Source: CAD feature listing. Evaluate the final solid. Frame: model axes, mm. Face numbers are marked on the shaded views. A direction names the side the tool comes from. Give positions to 0.01 mm unless a question says otherwise; leave off trailing zeros. Loops run counter-clockwise (first coordinate to the right, second up) from the corner with the lowest first, then second, coordinate; pieces in that order, holes last. Notation, with made-up numbers: (89, 78.5) -> (108, 78.5) arc R15 cw to (108, 105.5) -> close; hole circle Ø2 at (75, -4). An arc over 180 degrees is marked (long way). Answer as a JSON object with one key per item and string values. Group by question number.
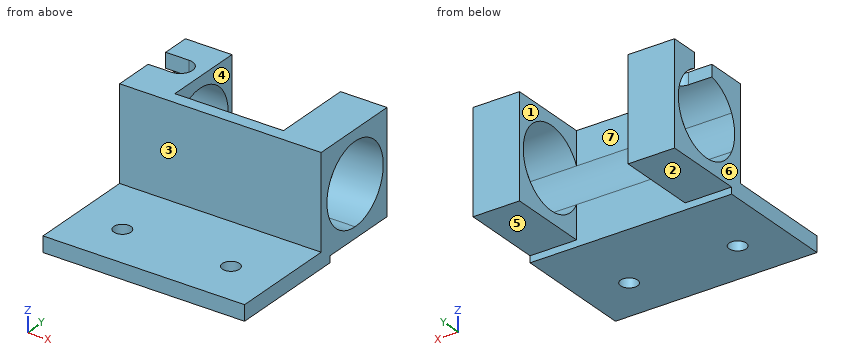
from build123d import *

# Parameters (mm, degrees)
CROQUIS2_W              = 65
CROQUIS2_H              = 35
CROQUIS2_R              = 2.75
SALIENTE_EXTRUIR1_DEPTH = 5
CROQUIS3_W              = 65
CROQUIS3_H              = 35
SALIENTE_EXTRUIR2_DEPTH = 4
SALIENTE_EXTRUIR3_DEPTH = 15
SALIENTE_EXTRUIR4_START = -65
SALIENTE_EXTRUIR4_DEPTH = 15
CORTAR_EXTRUIR1_DEPTH   = 85.965620518
CORTAR_EXTRUIR2_START   = -32.882450487
CORTAR_EXTRUIR2_DEPTH   = 4.823037372


# Read off the part's stored shape, not the designer's step: Cortar-Extruir2
with BuildPart() as part:
    # Croquis2 → Saliente-Extruir1 (new body)
    with BuildSketch(Plane.XY):
        with Locations((0, -5.5)):
            Rectangle(CROQUIS2_W, CROQUIS2_H)
        with Locations((17.5, -8)):
            Circle(CROQUIS2_R, mode=Mode.SUBTRACT)
        with Locations((-17.5, -8)):
            Circle(CROQUIS2_R, mode=Mode.SUBTRACT)
    extrude(amount=SALIENTE_EXTRUIR1_DEPTH)

    # Croquis3 → Saliente-Extruir2 (add)
    with BuildSketch(Plane(origin=(0, 12, 0), x_dir=(1, 0, 0), z_dir=(0, 1, 0))):
        with Locations((0, -17.5)):
            Rectangle(CROQUIS3_W, CROQUIS3_H)
    extrude(amount=SALIENTE_EXTRUIR2_DEPTH)

    # Croquis4 → Saliente-Extruir3 (add)
    with BuildSketch(Plane(origin=(32.5, 0, 0), x_dir=(0, 0, -1), z_dir=(1, 0, 0))):
        with BuildLine():
            Line((-35, 42.06134413), (-35, 16))
            Line((-35, 16), (-24.382874813, 16))
            ThreePointArc((-24.382874813, 16), (-25.295997358, 38.453973796), (-5.683774756, 27.482398858))
            ThreePointArc((-5.683774756, 27.482398858), (-7.587199819, 20.745176256), (-12.7346747, 16))
            Line((-12.7346747, 16), (-2.117549513, 16))
            Line((-2.117549513, 16), (-2.117549513, 42.06134413))
            Line((-2.117549513, 42.06134413), (-35, 42.06134413))
        make_face()
        with BuildLine():
            Line((-12.7346747, 16), (-24.382874813, 16))
            ThreePointArc((-24.382874813, 16), (-18.558774756, 14.607398858), (-12.7346747, 16))
        make_face()
        with BuildLine():
            ThreePointArc((-5.683774756, 27.482398858), (-25.295997358, 38.453973796), (-24.382874813, 16))
            Line((-24.382874813, 16), (-12.7346747, 16))
            ThreePointArc((-12.7346747, 16), (-7.587199819, 20.745176256), (-5.683774756, 27.482398858))
        make_face()
    extrude(amount=-SALIENTE_EXTRUIR3_DEPTH)

    # Croquis4<6> → Saliente-Extruir4 (add)
    with BuildSketch(Plane(origin=(32.5, 0, 0), x_dir=(0, 0, -1), z_dir=(1, 0, 0)).offset(SALIENTE_EXTRUIR4_START)):
        with BuildLine():
            Line((-35, 42.06134413), (-35, 16))
            Line((-35, 16), (-24.382874813, 16))
            ThreePointArc((-24.382874813, 16), (-25.295997358, 38.453973796), (-5.683774756, 27.482398858))
            ThreePointArc((-5.683774756, 27.482398858), (-7.587199819, 20.745176256), (-12.7346747, 16))
            Line((-12.7346747, 16), (-2.117549513, 16))
            Line((-2.117549513, 16), (-2.117549513, 42.06134413))
            Line((-2.117549513, 42.06134413), (-35, 42.06134413))
        make_face()
        with BuildLine():
            Line((-12.7346747, 16), (-24.382874813, 16))
            ThreePointArc((-24.382874813, 16), (-18.558774756, 14.607398858), (-12.7346747, 16))
        make_face()
        with BuildLine():
            ThreePointArc((-5.683774756, 27.482398858), (-25.295997358, 38.453973796), (-24.382874813, 16))
            Line((-24.382874813, 16), (-12.7346747, 16))
            ThreePointArc((-12.7346747, 16), (-7.587199819, 20.745176256), (-5.683774756, 27.482398858))
        make_face()
    extrude(amount=SALIENTE_EXTRUIR4_DEPTH)

    # Croquis4<4> → Cortar-Extruir1 (cut, through all)
    with BuildSketch(Plane(origin=(32.5, 0, 0), x_dir=(0, 0, -1), z_dir=(1, 0, 0))):
        with BuildLine():
            Line((-12.7346747, 16), (-24.382874813, 16))
            ThreePointArc((-24.382874813, 16), (-18.558774756, 14.607398858), (-12.7346747, 16))
        make_face()
        with BuildLine():
            ThreePointArc((-5.683774756, 27.482398858), (-25.295997358, 38.453973796), (-24.382874813, 16))
            Line((-24.382874813, 16), (-12.7346747, 16))
            ThreePointArc((-12.7346747, 16), (-7.587199819, 20.745176256), (-5.683774756, 27.482398858))
        make_face()
    extrude(amount=-CORTAR_EXTRUIR1_DEPTH, mode=Mode.SUBTRACT)

    # Cortar-Extruir2 outline → Cortar-Extruir2 (cut)
    with BuildSketch(Plane(origin=(0, 0, 2.117549513), x_dir=(-1, 0, 0), z_dir=(0, 0, -1)).offset(CORTAR_EXTRUIR2_START)):
        with BuildLine():
            Line((32.5, 33.030672065), (25, 33.030672065))
            ThreePointArc((25, 33.030672065), (21, 29.030672065), (25, 25.030672065))
            Line((25, 25.030672065), (32.5, 25.030672065))
            Line((32.5, 25.030672065), (32.5, 33.030672065))
        make_face()
    extrude(amount=CORTAR_EXTRUIR2_DEPTH, mode=Mode.SUBTRACT)


solid = part.part
(1) Material intervals for line 1 (X direction, y = 16.5, z = 31.5); line 2 (Z direction, x = -8, y = 5); line 3 (Y direction, x = 0, z = 25), sorted ascending. Write a range as from..to.
(2) Mould query, pull axis X, two halves, no side actions, for the marked faces 4, 5, 6 and 7. Classes: pulls with the +X half, pulls with the -X half, needs draft (parallel to the pull), parting line crosses it, or undercut.
(3) Section query B-B on x = 25.5. Return the cut outline in (y, z) (3 decimals).
(4) Section query A-A on y = -8. Return the cut outline in (x, z), plus the area to 3 significant figures.
(5) First-contact query: pin 1 (12 mm diameter, centred on y = -12.5, z = 15, fed in from -X); pin 2 (1.5 mm diameter, centred on x = 25.5, y = 7, fed in from -Z); pin 3 (15 mm diameter, centred on x = 13, z = 23.5, fed in from -Y); pin 4 (17.5 mm diameter, centred on x = 0.5, y = -1.5, fed in from +Z). Flat tips, straight axial feed; report the tip coordinate or a pass-through.
(6) Section query D-D on y = 36. Return the cut outline in (x, z).
(7) Section query C-C on x = -13. Return the cut outline in (y, z) (3 decimals).
(8) Access query for the marked faces 1, 2 and 3. Directions: +Z, -Z, +X, -X, +Y, -Y. A direction counts if a zero-diameter tool reaches every point of the face in a straight line with its end or side. Return the directions, or none.
Result:
{
 "1": {"line 1": "-32.5..-17.5, 17.5..32.5", "line 2": "0..5", "line 3": "12..16"},
 "2": {"face 4": "undercut", "face 5": "needs draft", "face 6": "pulls with the -X half", "face 7": "undercut"},
 "3": {"outline": "(-23, 0) -> (16, 0) -> (16, 2.118) -> (42.061, 2.118) -> (42.061, 35) -> (12, 35) -> (12, 5) -> (-23, 5) -> close; hole circle Ø25.75 at (27.482, 18.559)"},
 "4": {"outline": "(-32.5, 0) -> (-20.25, 0) -> (-20.25, 5) -> (-32.5, 5) -> close; (-14.75, 0) -> (14.75, 0) -> (14.75, 5) -> (-14.75, 5) -> close; (20.25, 0) -> (32.5, 0) -> (32.5, 5) -> (20.25, 5) -> close", "area": "270 mm²"},
 "5": {"pin 1": "through", "pin 2": "z = 0", "pin 3": "y = 12", "pin 4": "z = 5"},
 "6": {"outline": "(-32.5, 2.12) -> (-17.5, 2.12) -> (-17.5, 8.9) -> (-32.5, 8.9) -> close; (-32.5, 28.21) -> (-17.5, 28.21) -> (-17.5, 35) -> (-32.5, 35) -> close; (17.5, 2.12) -> (32.5, 2.12) -> (32.5, 8.9) -> (17.5, 8.9) -> close; (17.5, 28.21) -> (32.5, 28.21) -> (32.5, 35) -> (17.5, 35) -> close"},
 "7": {"outline": "(-23, 0) -> (16, 0) -> (16, 12.735) arc R12.875 cw to (16, 24.383) -> (16, 35) -> (12, 35) -> (12, 5) -> (-23, 5) -> close"},
 "8": {"face 1": "+Z, -Z, +Y", "face 2": "-Z, +X, -X, +Y", "face 3": "+Z, +X, -X, -Y"}
}
